Can you work these out from the model? Positions are in its coordinate system, mm. A direction names the side the tool comes from. Give positions to 0.01 mm unless a question says otherwise; leave off trailing zeros. Write each loop counter-clockwise with the first axis right and the second up, starting at its lowest first coordinate (ties: lowest second). Pieces come first, ordered by that corner, then holes.
from build123d import *

# Parameters (mm, degrees)
BOSS_EXTRUDE1_DEPTH = 10
SKETCH2_OUTSIDE_W   = 47.032
SKETCH2_OUTSIDE_H   = 47.728
SKETCH2_OUTSIDE_R   = 2.25
CUT_EXTRUDE1_DEPTH  = 11
CUT_EXTRUDE1_TAPER  = 60
SKETCH3_OUTSIDE_W   = 47.032
SKETCH3_OUTSIDE_H   = 47.728
SKETCH3_OUTSIDE_R   = 2.25
CUT_EXTRUDE2_DEPTH  = 11
CUT_EXTRUDE2_TAPER  = 60
SKETCH4_R           = 1.25
CUT_EXTRUDE3_DEPTH  = 4.8
SKETCH5_R           = 1.25
BOSS_EXTRUDE2_DEPTH = 3.9
CHAMFER1_SIZE       = 0.36
CHAMFER1_SIZE2      = 0.429031293


with BuildPart() as part:
    # Sketch1 → Boss-Extrude1 (new body)
    with BuildSketch(Plane(origin=(0, 0, 0), x_dir=(1, 0, 0), z_dir=(0, 1, 0))):
        Polygon((0, 2.598076211), (-2.25, 1.299038106), (-2.25, -1.299038106), (0, -2.598076211), (2.25, -1.299038106), (2.25, 1.299038106), align=None)
    extrude(amount=BOSS_EXTRUDE1_DEPTH)

    # Sketch2 outside → Cut-Extrude1 (cut, through all)
    with BuildSketch(Plane(origin=(0, 10, 0), x_dir=(1, 0, 0), z_dir=(0, 1, 0))):
        Rectangle(SKETCH2_OUTSIDE_W, SKETCH2_OUTSIDE_H)
        Circle(SKETCH2_OUTSIDE_R, mode=Mode.SUBTRACT)
    extrude(amount=-CUT_EXTRUDE1_DEPTH, taper=CUT_EXTRUDE1_TAPER, mode=Mode.SUBTRACT)

    # Sketch3 outside → Cut-Extrude2 (cut, through all)
    with BuildSketch(Plane.XZ):
        Rectangle(SKETCH3_OUTSIDE_W, SKETCH3_OUTSIDE_H)
        Circle(SKETCH3_OUTSIDE_R, mode=Mode.SUBTRACT)
    extrude(amount=-CUT_EXTRUDE2_DEPTH, taper=CUT_EXTRUDE2_TAPER, mode=Mode.SUBTRACT)

    # Sketch4 → Cut-Extrude3 (cut)
    with BuildSketch(Plane(origin=(0, 10, 0), x_dir=(1, 0, 0), z_dir=(0, 1, 0))):
        Circle(SKETCH4_R)
    extrude(amount=-CUT_EXTRUDE3_DEPTH, mode=Mode.SUBTRACT)

    # Sketch5 → Boss-Extrude2 (add)
    with BuildSketch(Plane.XZ):
        Circle(SKETCH5_R)
    extrude(amount=BOSS_EXTRUDE2_DEPTH)

    # Chamfer1
    chamfer1_edges = [part.edges().sort_by_distance(p)[0] for p in [
        (-1.25, -3.9, 0),
    ]]
    chamfer1_side = [part.faces().sort_by_distance(p)[0] for p in [
        (-1.25, -1.95, 0),
    ]]
    chamfer(chamfer1_edges, length=CHAMFER1_SIZE, length2=CHAMFER1_SIZE2, reference=chamfer1_side[0])


solid = part.part
(1) For faces 1 (the face through (1, 10, 1)), 2 (the face through (1, 0, 1)), which set-ups out of +Z, -Z, +X, -X, +Y, -Y let a thin tool reach every point of the face, with its end or its side?
Returned:
face 1: +Z, -Z, +X, -X, +Y
face 2: -Y
(2) If I drill on L1, parallel to X at y = 6.3, z = 0; L2, parallel to Y at x = -1.45, z = 1.4; L3, parallel to Y at x = -0.7, z = 0.2, over which ranges is the centre line in solid material (lowest first)?
Returned:
L1: x = -2.25 to -1.25, 1.25 to 2.25
L2: y = 0 to 10
L3: y = -3.9 to 5.2
(3) Imagine slicing it at B-B, the plane y = -1.75. Write out the boundary of the cut face in (x, z), plus the area to 3 significant figures.
Returned:
outline: circle Ø2.5 at (0, 0)
area: 4.91 mm2
(4) If we mould it in two halves opening along Z, with no side actions, what happens to faces 3 (the face through (1.109, 4.93, 1.958)), 4 (the face through (-0.27, 7.63, 1.22)), 5 (the face through (-0.27, -1.75, -1.22))? For each: +Z half, -Z half, draft (parallel to the pull), parting line (faces both ways), or undercut.
Returned:
face 3: +Z half
face 4: undercut
face 5: parting line
(5) Imagine slicing it at A-A, the plane y = 5.75. Write out the boundary of the cut face in (x, z), plus the area to 3 significant figures.
Returned:
outline: (-2.25, -1.3) - (0, -2.6) - (2.25, -1.3) - (2.25, 1.3) - (0, 2.6) - (-2.25, 1.3) - close; hole circle Ø2.5 at (0, 0)
area: 12.6 mm2
(6) Will these pins go through, and if not, where does the flat tip stop? P1, Ø1, axis at x = -0.5, z = -2, coming from the -Y side; P2, Ø1.2, axis at x = 0, z = 0, coming from the +Y side.
Returned:
P1: stops at y = 0
P2: stops at y = 5.2
